Source: CAD feature listing. Evaluate the final solid. Frame: model axes, mm. A direction names the side the tool comes from. Give positions to 0.01 mm unless a question says otherwise; leave off trailing zeros. Order: outer loops, then holes, each group sorted by start corner. A loop starts at its lowest first (then second) coordinate and runs counter-clockwise, first axis right, second up.
from build123d import *

# Parameters (mm, degrees)
F0_R     = 12.5
F1_DEPTH = 82.5
F3_DEPTH = 120
F4_R     = 8
F5_R     = 6
F6_DEPTH = 25


with BuildPart() as f1:
    # F0 (on Front) → F1 (new body, symmetric)
    with BuildSketch(Plane.XZ):
        Circle(F0_R)
    extrude(amount=F1_DEPTH, both=True)

    # F2 (on face) → F3 (join)
    with BuildSketch(Plane(origin=(0, 82.5, 0), x_dir=(-1, 0, 0), z_dir=(0, 1, 0))):
        with BuildLine():
            Line((6.25, -10.825318), (6.25, 10.825318))
            ThreePointArc((6.25, 10.825318), (0, 12.5), (-6.25, 10.825318))
            Line((-6.25, 10.825318), (-6.25, -10.825318))
            ThreePointArc((-6.25, -10.825318), (0, -12.5), (6.25, -10.825318))
        make_face()
    extrude(amount=F3_DEPTH)

    # F4
    f4_edges = [f1.edges().sort_by_distance(p)[0] for p in [
        (-12.5, -82.5, 0),
    ]]
    fillet(f4_edges, radius=F4_R)

    # F5 (on face) → F6 (cut)
    with BuildSketch(Plane.YZ.offset(6.25)):
        with Locations((192.5, 0)):
            Circle(F5_R)
    extrude(amount=-F6_DEPTH, mode=Mode.SUBTRACT)


solid = f1.part
1) Section query B-B on y = -21. Output: boundary loops of the cut face in (x, z).
Checks:
outline: circle Ø25 at (0, 0)
2) Ray query, L1, parallel to X at y = 89.5, z = 0.75; L2, parallel to Z at x = -0.5, y = 192.5; L3, parallel to Z at x = 2, y = 192.5. Return the intervals inside material, ascending.
Checks:
L1: x = -6.25 to 6.25
L2: z = -12.49 to -6, 6 to 12.49
L3: z = -12.34 to -6, 6 to 12.34
3) Reachability of faces 1 (the face through (6.25, 142, 0)), 2 (the face through (0, 202.5, 0)) from +Z, -Z, +X, -X, +Y, -Y: full face, straight path, thin tool, end or side. Return the list, or none.
Checks:
face 1: +Z, -Z, +X, +Y
face 2: +Z, -Z, +X, -X, +Y
4) Section query A-A on y = 192.5. Output: boundary loops of the cut face in (x, z).
Checks:
outline: (-6.25, -10.83) arc R12.5 ccw to (6.25, -10.83) - (6.25, -6) - (-6.25, -6) - close; (-6.25, 6) - (6.25, 6) - (6.25, 10.83) arc R12.5 ccw to (-6.25, 10.83) - close
5) Section query C-C on y = 135. Output: boundary loops of the cut face in (x, z), and give its area (3 significant figures).
Checks:
outline: (-6.25, -10.83) arc R12.5 ccw to (6.25, -10.83) - (6.25, 10.83) arc R12.5 ccw to (-6.25, 10.83) - close
area: 299 mm2
6) Pull-direction query (Y, two-part tool) for faces 3 (the face through (-9, 82.5, 0)), 4 (the face through (0, -82.5, 0)), 5 (the face through (-6.25, 142, 0)), 6 (the face through (0.088, 186.506, 0.264)); classes: +Y half, -Y half, draft (parallel to the pull), parting line (faces both ways), or undercut.
Checks:
face 3: +Y half
face 4: -Y half
face 5: draft
face 6: undercut
7) First-contact query: pin 1 Ø5 at (x, z) = (10.5, 5.5) entering from +Y; pin 2 Ø11 at (y, z) = (128.5, 1) entering from -X; pin 3 Ø12 at (y, z) = (170, 9) entering from +X; pin 4 Ø12 at (y, z) = (-32, -3) entering from -X. Flat tips, straight axial feed; report the tip coordinate or a pass-through.
Checks:
pin 1: stops at y = 82.5
pin 2: stops at x = -6.25
pin 3: stops at x = 6.25
pin 4: stops at x = -12.5
